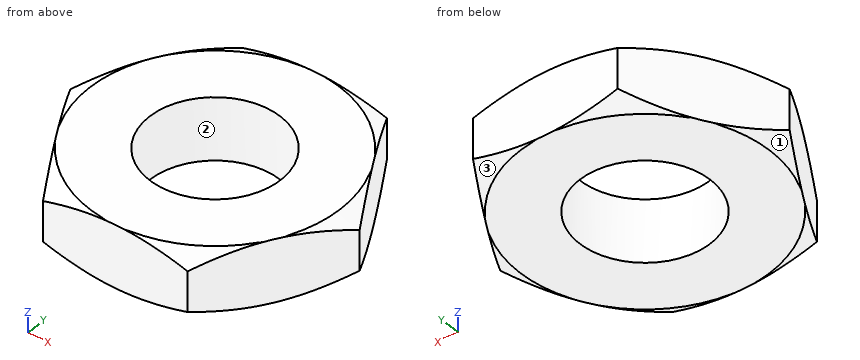
```python
from build123d import *

# Parameters (mm, degrees)
BOSS_EXTRUDE1_DEPTH = 3.25
M8_TAPPED_HOLE1_D   = 6.8


with BuildPart() as part:
    # Sketch1 → Boss-Extrude1 (new body)
    with BuildSketch(Plane.XY):
        Polygon((3.75277675, -6.5), (7.505553499, 0), (3.75277675, 6.5), (-3.75277675, 6.5), (-7.505553499, 0), (-3.75277675, -6.5), align=None)
    extrude(amount=BOSS_EXTRUDE1_DEPTH)

    # Sketch3 → Cut-Revolve1 (revolve, cut)
    with BuildSketch(Plane(origin=(0, 0, 0), x_dir=(0, 0, -1), z_dir=(1, 0, 0))):
        Polygon((-1.711637245, 9.464642673), (0, 6.5), (0, 9.464642673), align=None)
        Polygon((-3.25, 6.5), (-3.25, 7.969336789), (-2.401678009, 7.969336789), align=None)
    revolve(axis=Axis((0, 0, 0), (0, 0, -1)), mode=Mode.SUBTRACT)

    # M8 Tapped Hole1 (through all)
    with Locations(Plane.XY.offset(3.25)):
        with Locations((0, 0)):
            Hole(M8_TAPPED_HOLE1_D / 2)


solid = part.part
```
Source: CAD feature listing. Evaluate the final solid. Frame: model axes, mm. Face numbers are marked on the shaded views. Round coordinates to 2 decimals unless told otherwise and drop trailing zeros. Loops run counter-clockwise (first coordinate to the right, second up) from the corner with the lowest first, then second, coordinate; pieces in that order, holes last. Notation, with made-up numbers: M 12.5,-27.5 L 17.5,-27.5 A11 ccw 17.5,-8.5 Z; hole C -12.5,54 d11. An arc over 180 degrees is marked long. Use a Markdown table: item, result. Add a question column.
1. Line query: line 1 (Y direction, x = 0, z = 2.25); line 2 (Y direction, x = 0.75, z = 1.9); line 3 (X direction, y = 1.5, z = 2.9). Output: solid intervals per line, ascending.
2. Section query A-A on z = 0.75. Return the cut outline in (x, y).
3. Contact query for a flat-ended pin moving along its axis: P1, Ø1, axis at y = -3, z = 1.5, coming from the +X side. Output: stop coordinate, or through.
4. Mould query, pull axis X, two halves, no side actions, for the marked faces 1, 2 and 3. Classes: pulls with the +X half, pulls with the -X half, needs draft (parallel to the pull), parting line crosses it, or undercut.
Reported:
| question | item | result |
|---|---|---|
| 1 | line 1 | y = -6.5 to -3.4, 3.4 to 6.5 |
| 1 | line 2 | y = -6.5 to -3.32, 3.32 to 6.5 |
| 1 | line 3 | x = -6.64 to -3.05, 3.05 to 6.64 |
| 2 | outline | M -7.51,0 L -3.75,-6.5 L 3.75,-6.5 L 7.51,0 L 3.75,6.5 L -3.75,6.5 Z; hole C 0,0 d6.8 |
| 3 | P1 | stops at x = 6.06 |
| 4 | face 1 | pulls with the -X half |
| 4 | face 2 | undercut |
| 4 | face 3 | pulls with the +X half |
